Check sheet for the modelled part. Datum: model origin and axes. Units: mm. Face numbers are marked on the shaded views. A direction names the side the tool comes from. Round coordinates to 2 decimals unless told otherwise and drop trailing zeros. Loops run counter-clockwise (first coordinate to the right, second up) from the corner with the lowest first, then second, coordinate; pieces in that order, holes last. Notation, with made-up numbers: (43, 21) - (56, 21) arc R3 ccw to (56, 25) - close; hole circle Ø7 at (74, -40). An arc over 180 degrees is marked (long way). Answer in a Markdown table with one row per item. Add a question column.
(1) Access from +Z, -Z, +X, -X, +Y, -Y to the whole of each face (thin tool, end or side, straight path). Record for the marked faces 1, 2 and 3.
(2) Mould release check, pull along Y, two halves, no side actions. Record for the marked faces 4, 5 and 6: +Y half, -Y half, draft (parallel to the pull), parting line (faces both ways), or undercut.
(3) Cross-section at B-B on y = 60. Enter the section's corners in (x, z).
(4) Cross-section at D-D on y = 326.5. Enter the section's corners in (x, z).
(5) Cross-section at C-C on y = -98. Enter the section's corners in (x, z).
(6) Thickness scan on line 1 along X through (y, z) = (-89, 140); line 2 along Y through (x, z) = (69, 53.5); line 3 along Y through (x, z) = (-54, 245.5). Record the ranges inside material, lowest first.
(7) Cross-section at A-A on x = 0. Enter the section's corners in (y, z).
(8) Gauge pin test, flat ends, axial feed: pin 1 (5 mm diameter, centred on x = 49.5, y = 406, fed in from +Z); pin 2 (5 mm diameter, centred on x = -30, y = 455, fed in from -Z). Record the tip position at first contact, or that the pin passes through.
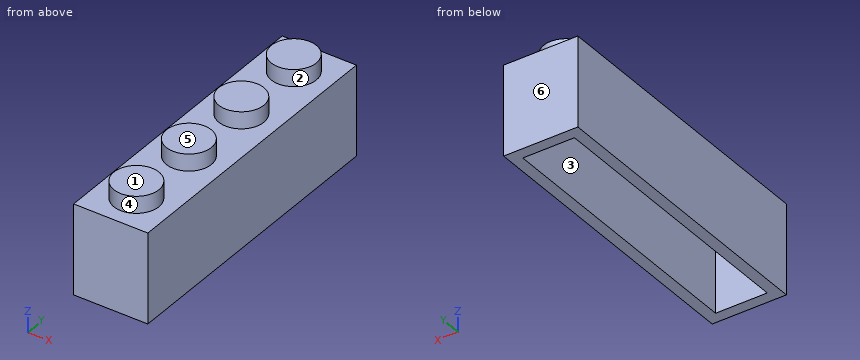
from build123d import *

# Parameters (mm, degrees)
F0_W     = 200.66
F0_H     = 807.72
F1_DEPTH = 243.84
F2_R     = 60.96
F3_DEPTH = 45.72
F4_W     = 139.7
F4_H     = 746.76
F5_DEPTH = 213.36


with BuildPart() as f1:
    # F0 (on Top) → F1 (new body)
    with BuildSketch(Plane.XY):
        with Locations((-0.261474, 252.359729)):
            Rectangle(F0_W, F0_H)
    extrude(amount=F1_DEPTH)

    # F2 (on face) → F3 (join)
    with BuildSketch(Plane.XY.offset(243.84)):
        with Locations((0, -52.440616)):
            Circle(F2_R)
        with Locations((0, 150.759384)):
            Circle(F2_R)
        with Locations((0, 353.959384)):
            Circle(F2_R)
        with Locations((0, 557.159384)):
            Circle(F2_R)
    extrude(amount=F3_DEPTH)

    # F4 (on face) → F5 (cut)
    with BuildSketch(Plane(origin=(0, 0, 0), x_dir=(1, 0, 0), z_dir=(0, 0, -1))):
        with Locations((-0.261474, -252.359729)):
            Rectangle(F4_W, F4_H)
    extrude(amount=-F5_DEPTH, mode=Mode.SUBTRACT)


solid = f1.part
Answers:
| question | item | result |
|---|---|---|
| 1 | face 1 | +Z, +X, -X, +Y, -Y |
| 1 | face 2 | +Z |
| 1 | face 3 | -Z |
| 2 | face 4 | undercut |
| 2 | face 5 | draft |
| 2 | face 6 | +Y half |
| 3 | outline | (-100.59, 0) - (-70.11, 0) - (-70.11, 213.36) - (69.59, 213.36) - (69.59, 0) - (100.07, 0) - (100.07, 243.84) - (-100.59, 243.84) - close |
| 4 | outline | (-100.59, 0) - (-70.11, 0) - (-70.11, 213.36) - (69.59, 213.36) - (69.59, 0) - (100.07, 0) - (100.07, 243.84) - (54.43, 243.84) - (54.43, 289.56) - (-54.43, 289.56) - (-54.43, 243.84) - (-100.59, 243.84) - close |
| 5 | outline | (-100.59, 0) - (-70.11, 0) - (-70.11, 213.36) - (69.59, 213.36) - (69.59, 0) - (100.07, 0) - (100.07, 243.84) - (40.5, 243.84) - (40.5, 289.56) - (-40.5, 289.56) - (-40.5, 243.84) - (-100.59, 243.84) - close |
| 6 | line 1 | x = -100.59 to -70.11, 69.59 to 100.07 |
| 6 | line 2 | y = -151.5 to -121.02, 625.74 to 656.22 |
| 6 | line 3 | y = -80.73 to -24.15, 122.47 to 179.05, 325.67 to 382.25, 528.87 to 585.45 |
| 7 | outline | (-151.5, 0) - (-121.02, 0) - (-121.02, 213.36) - (625.74, 213.36) - (625.74, 0) - (656.22, 0) - (656.22, 243.84) - (618.12, 243.84) - (618.12, 289.56) - (496.2, 289.56) - (496.2, 243.84) - (414.92, 243.84) - (414.92, 289.56) - (293, 289.56) - (293, 243.84) - (211.72, 243.84) - (211.72, 289.56) - (89.8, 289.56) - (89.8, 243.84) - (8.52, 243.84) - (8.52, 289.56) - (-113.4, 289.56) - (-113.4, 243.84) - (-151.5, 243.84) - close |
| 8 | pin 1 | stops at z = 243.84 |
| 8 | pin 2 | stops at z = 213.36 |
